Could you check a few things on this model? Use its own coordinates, in mm. A direction names the side the tool comes from. Give positions to 0.01 mm unless a question says otherwise; leave off trailing zeros. Write each loop counter-clockwise with the first axis right and the second up, starting at its lowest first coordinate (ties: lowest second). Pieces come first, ordered by that corner, then holes. Notation, with made-up numbers: (56.5, -36.5) -> (91.5, -36.5) arc R21 ccw to (91.5, -1.5) -> close; hole circle Ø7 at (64.5, 80.5). An arc over 180 degrees is marked (long way). One line per question, with ' | ' between items.
from build123d import *

# Parameters (mm, degrees)
F0_W     = 44.45
F0_H     = 31.75
F1_DEPTH = 50.8
F3_SIZE2 = 6.35
F3_SIZE  = 6.35
F4_R     = 6.35
F5_D     = 11.50874
F5_DEPTH = 25.4
F5_TIP   = 3.4575743203


with BuildPart() as f1:
    # F0 (on Front) → F1 (new body)
    with BuildSketch(Plane.XZ):
        with Locations((22.225, 15.875)):
            Rectangle(F0_W, F0_H)
    extrude(amount=F1_DEPTH)

    # F3
    f3_edges = [f1.edges().sort_by_distance(p)[0] for p in [
        (0, -25.4, 31.75),
        (22.225, -50.8, 31.75),
        (44.45, -25.4, 31.75),
        (22.225, 0, 31.75),
    ]]
    chamfer(f3_edges, length=F3_SIZE, length2=F3_SIZE2)

    # F4
    f4_edges = [f1.edges().sort_by_distance(p)[0] for p in [
        (41.275, -47.625, 28.575),
        (41.275, -3.175, 28.575),
        (3.175, -3.175, 28.575),
        (3.175, -47.625, 28.575),
    ]]
    fillet(f4_edges, radius=F4_R)

    # F5
    with Locations(Plane.XY.offset(31.75)):
        with Locations((22.225, -25.4)):
            Hole(F5_D / 2, depth=F5_DEPTH)
            with Locations((0, 0, -(F5_DEPTH + F5_TIP / 2))):  # 118° drill point
                Cone(0, F5_D / 2, F5_TIP, mode=Mode.SUBTRACT)


solid = f1.part
Q1. Imagine slicing it at B-B on y = -15. Please give me the cut outline in (x, z).
Answer below:
outline: (0, 0) -> (44.45, 0) -> (44.45, 25.4) -> (38.1, 31.75) -> (6.35, 31.75) -> (0, 25.4) -> close
Q2. Imagine slicing it at D-D on z = 5. Please give me the cut outline in (x, y) (3 decimals), and give its area (3 significant figures).
Answer below:
outline: (0, -50.8) -> (44.45, -50.8) -> (44.45, 0) -> (0, 0) -> close; hole circle Ø7.015 at (22.225, -25.4) | area: 2,220 mm^2
Q3. Imagine slicing it at C-C on x = 29. Please give me the cut outline in (y, z), and give its area (3 significant figures).
Answer below:
outline: (-50.8, 0) -> (0, 0) -> (0, 25.4) -> (-6.35, 31.75) -> (-44.45, 31.75) -> (-50.8, 25.4) -> close | area: 1,570 mm^2
Q4. If I drill on line 1 along X through (y, z) = (-25, 17); line 2 along Y through (x, z) = (23, 19.5); line 3 along X through (y, z) = (-27, 25.5), over which ranges is the centre line in solid material (lowest first)?
Answer below:
line 1: x = 0 to 16.48, 27.97 to 44.45 | line 2: y = -50.8 to -31.1, -19.7 to 0 | line 3: x = 0.1 to 16.7, 27.75 to 44.35
Q5. On a 3-axis mill with a long thin cutter (end or side, diameter ignored), from which of +Z, -Z, +X, -X, +Y, -Y can I reach the whole of each face in a straight line? I mean faces 1 (the flat face through (22, 0, 13)), 2 (the cylindrical face through (26.466, -21.511, 18.872)). Say none if no direction works.
Answer below:
face 1: +Z, -Z, +X, -X, +Y | face 2: +Z
Q6. If we mould it in two halves opening along X, with no side actions, what happens to faces 3 (the flat face through (22, -25, 0)), 4 (the conical face through (22.686, -26.287, 3.493)), 5 (the flat face through (0, -25, 13))? For each: +X half, -X half, draft (parallel to the pull), parting line (faces both ways), or undercut.
Answer below:
face 3: draft | face 4: undercut | face 5: -X half
Q7. Will these pins go through, and if not, where does the flat tip stop? pin 1 (1 mm diameter, centred on x = 25, y = -28, fed in from +Z); pin 2 (2 mm diameter, centred on x = 10, z = 27.5, fed in from +Y).
Answer below:
pin 1: stops at z = 5.48 | pin 2: stops at y = -1.1
Q8. Imagine slicing it at A-A on z = 21. Please give me the cut outline in (x, y) (3 decimals).
Answer below:
outline: (0, -50.8) -> (44.45, -50.8) -> (44.45, 0) -> (0, 0) -> close; hole circle Ø11.509 at (22.225, -25.4)
